from build123d import *

# Parameters (mm, degrees)
ESQUISSE1_W             = 112
ESQUISSE1_H             = 150
BOSS_EXTRU_1_DEPTH      = 3.5
ENL_V_MAT_EXTRU_1_REACH = 5.5
ESQUISSE2_R             = 2.5


with BuildPart() as part:
    # Esquisse1 → Boss.-Extru.1 (new body)
    with BuildSketch(Plane(origin=(0, 0, 0), x_dir=(1, 0, 0), z_dir=(0, 1, 0))):
        Rectangle(ESQUISSE1_W, ESQUISSE1_H)
    extrude(amount=BOSS_EXTRU_1_DEPTH)

    # Esquisse2 → Enlèv. mat.-Extru.1 (cut, up to next)
    with BuildSketch(Plane(origin=(0, 3.5, 0), x_dir=(1, 0, 0), z_dir=(0, 1, 0)), mode=Mode.PRIVATE) as enl_v_mat_extru_1_sk1:
        with Locations((51.5, 67.5)):
            Circle(ESQUISSE2_R)
    enl_v_mat_extru_1_tool1 = extrude(enl_v_mat_extru_1_sk1.sketch, amount=-ENL_V_MAT_EXTRU_1_REACH, mode=Mode.PRIVATE) & part.part
    add(enl_v_mat_extru_1_tool1.solids().sort_by_distance((51.5, 3.5, -67.5))[0], mode=Mode.SUBTRACT)
    # Esquisse2 → Enlèv. mat.-Extru.1 (cut, up to next)
    with BuildSketch(Plane(origin=(0, 3.5, 0), x_dir=(1, 0, 0), z_dir=(0, 1, 0)), mode=Mode.PRIVATE) as enl_v_mat_extru_1_sk2:
        with Locations((-51.5, 47.5)):
            Circle(ESQUISSE2_R)
    enl_v_mat_extru_1_tool2 = extrude(enl_v_mat_extru_1_sk2.sketch, amount=-ENL_V_MAT_EXTRU_1_REACH, mode=Mode.PRIVATE) & part.part
    add(enl_v_mat_extru_1_tool2.solids().sort_by_distance((-51.5, 3.5, -47.5))[0], mode=Mode.SUBTRACT)
    # Esquisse2 → Enlèv. mat.-Extru.1 (cut, up to next)
    with BuildSketch(Plane(origin=(0, 3.5, 0), x_dir=(1, 0, 0), z_dir=(0, 1, 0)), mode=Mode.PRIVATE) as enl_v_mat_extru_1_sk3:
        with Locations((51.5, -37.5)):
            Circle(ESQUISSE2_R)
    enl_v_mat_extru_1_tool3 = extrude(enl_v_mat_extru_1_sk3.sketch, amount=-ENL_V_MAT_EXTRU_1_REACH, mode=Mode.PRIVATE) & part.part
    add(enl_v_mat_extru_1_tool3.solids().sort_by_distance((51.5, 3.5, 37.5))[0], mode=Mode.SUBTRACT)
    # Esquisse2 → Enlèv. mat.-Extru.1 (cut, up to next)
    with BuildSketch(Plane(origin=(0, 3.5, 0), x_dir=(1, 0, 0), z_dir=(0, 1, 0)), mode=Mode.PRIVATE) as enl_v_mat_extru_1_sk4:
        with Locations((-51.5, -57.5)):
            Circle(ESQUISSE2_R)
    enl_v_mat_extru_1_tool4 = extrude(enl_v_mat_extru_1_sk4.sketch, amount=-ENL_V_MAT_EXTRU_1_REACH, mode=Mode.PRIVATE) & part.part
    add(enl_v_mat_extru_1_tool4.solids().sort_by_distance((-51.5, 3.5, 57.5))[0], mode=Mode.SUBTRACT)


solid = part.part
The listing builds one solid part. Answer for the finished solid, in the listing's coordinates (mm). Give positions to 0.01 mm unless a question says otherwise; leave off trailing zeros. Order: outer loops, then holes, each group sorted by start corner. A loop starts at its lowest first (then second) coordinate and runs counter-clockwise, first axis right, second up. Notation, with made-up numbers: (-37.5, 63) - (-6.5, 63) arc R17 cw to (-6.5, 69) - close; hole circle Ø6 at (37, 24.5). An arc over 180 degrees is marked (long way). One line per item, written item: value. Start each with the question number.
1) A cutting plane is placed at B-B on z = 57.5. Give the vertices of the cut face in (x, y), then the cut area to 4 significant figures.
2) The mould has two halves that part along Z. Classify faces 1 (the face through (-1, 2, 75)), 2 (the face through (53.81, 1.77, 38.46)), 3 (the face through (-1, 3.5, -1)): released by +Z, released by -Z, zero draft, split by the parting line, or undercut.
3) Find the intervals of material crossed by L1, parallel to Z at x = -51.5, y = 1.1; L2, parallel to X at y = 0.7, z = 57.5; L3, parallel to X at y = 2.15, z = 37.5, in increasing order.
4) Given pin 1 Ø3 at (x, z) = (51.5, 37.5) entering from -Y, flat-ended and moving along its own axis, determine where the tip first touches the part or whether it passes through.
5) A cutting plane is placed at A-A on x = -51.5. Give the vertices of the cut face in (y, z), then the cut area to 3 significant figures.
Answer sheet:
1. outline: (-56, 0) - (-54, 0) - (-54, 3.5) - (-56, 3.5) - close; (-49, 0) - (56, 0) - (56, 3.5) - (-49, 3.5) - close
1. area: 374.5 mm2
2. face 1: released by +Z
2. face 2: undercut
2. face 3: zero draft
3. L1: z = -75 to -50, -45 to 55, 60 to 75
3. L2: x = -56 to -54, -49 to 56
3. L3: x = -56 to 49, 54 to 56
4. pin 1: passes through
5. outline: (0, -75) - (3.5, -75) - (3.5, -50) - (0, -50) - close; (0, -45) - (3.5, -45) - (3.5, 55) - (0, 55) - close; (0, 60) - (3.5, 60) - (3.5, 75) - (0, 75) - close
5. area: 490 mm2
